```python
from build123d import *

# Parameters (mm, degrees)
SKETCH1_W                      = 68
SKETCH1_H                      = 68
SKETCH1_R                      = 14.29
BOSS_EXTRUDE1_DEPTH            = 10
M6_CLEARANCE_HOLE1_D           = 6.6
M6_CLEARANCE_HOLE1_CSINK_D     = 6.65
M6_CLEARANCE_HOLE1_CSINK_ANGLE = 100
SKETCH5_W                      = 120
SKETCH5_H                      = 10
BOSS_EXTRUDE3_DEPTH            = 68
M6_CLEARANCE_HOLE2_D           = 6.6
M6_CLEARANCE_HOLE2_CSINK_D     = 6.65
M6_CLEARANCE_HOLE2_CSINK_ANGLE = 100


with BuildPart() as part:
    # Sketch1 → Boss-Extrude1 (new body)
    with BuildSketch(Plane.XY):
        Rectangle(SKETCH1_W, SKETCH1_H)
        Circle(SKETCH1_R, mode=Mode.SUBTRACT)
    extrude(amount=BOSS_EXTRUDE1_DEPTH)

    # M6 Clearance Hole1 (through all)
    with Locations(Plane(origin=(0, 0, 0), x_dir=(-1, 0, 0), z_dir=(0, 0, -1))):
        with Locations((-18.768735293, 18.768735293), (18.768735293, 18.768735293), (-18.768735293, -18.768735293), (18.768735293, -18.768735293)):
            CounterSinkHole(M6_CLEARANCE_HOLE1_D / 2, M6_CLEARANCE_HOLE1_CSINK_D / 2, counter_sink_angle=M6_CLEARANCE_HOLE1_CSINK_ANGLE)

    # Sketch5 → Boss-Extrude3 (add)
    with BuildSketch(Plane.XY.offset(10)):
        with Locations((0, 29)):
            Rectangle(SKETCH5_W, SKETCH5_H)
    extrude(amount=BOSS_EXTRUDE3_DEPTH)

    # M6 Clearance Hole2 (through all)
    with Locations(Plane(origin=(0, 34, 0), x_dir=(1, 0, 0), z_dir=(0, 1, 0))):
        with Locations((-30, -24), (30, -24), (-30, -64), (30, -64)):
            CounterSinkHole(M6_CLEARANCE_HOLE2_D / 2, M6_CLEARANCE_HOLE2_CSINK_D / 2, counter_sink_angle=M6_CLEARANCE_HOLE2_CSINK_ANGLE)


solid = part.part
```
The listing builds one solid part. Answer for the finished solid, in the listing's coordinates (mm). A direction names the side the tool comes from. Round coordinates to 2 decimals unless told otherwise and drop trailing zeros. Loops run counter-clockwise (first coordinate to the right, second up) from the corner with the lowest first, then second, coordinate; pieces in that order, holes last. Notation, with made-up numbers: (65.5, 40.5) - (120.5, 40.5) arc R16 cw to (120.5, 50.5) - close; hole circle Ø11 at (34.25, 19). An arc over 180 degrees is marked (long way). Use one line per item in the form item = value. Start each with the question number.
1. The part is cut by section C-C on x = 0. Determine the outline of the cut face in (y, z).
2. The part is cut by section A-A on z = 24. Determine the outline of the cut face in (x, y) (3 decimals), then the cut area to 3 significant figures.
3. For a pull along X with two mould halves and no side action, classify faces 1 (the face through (28.226, 28.92, 61.217)), 2 (the face through (-1, 29, 78)), 3 (the face through (-60, 29, 44)) as pulls with the +X half, pulls with the -X half, needs draft (parallel to the pull), parting line crosses it, or undercut.
4. Given pin 1 Ø3 at (x, z) = (-15, 68.5) entering from -Y; pin 2 Ø4 at (x, z) = (-30, 24) entering from +Y; pin 3 Ø10 at (x, y) = (12, 6) entering from +Z; pin 4 Ø8 at (y, z) = (-12.5, 6.5) entering from +X, each flat-ended and moving along its own axis, determine where each tip first touches the part or whether it passes through.
5. Consider line 1 (Z direction, x = -30, y = 30.5); line 2 (X direction, y = 29.5, z = 24); line 3 (Y direction, x = -6, z = 37). Determine where each line is inside the solid, lowest interval first. Write a range as [from, to].
6. A tool of negligible diameter and unlimited length cuts with its end or side. For faces 4 (the face through (47, 29, 10)), 5 (the face through (15.47, 18.91, 5.08)), 6 (the face through (0, -17, 10)), 7 (the face through (0, -34, 5)), 8 (the face through (-47, 29, 10)), from which of +Z, -Z, +X, -X, +Y, -Y can it reach the whole face along a straight path? Write none if from no direction.
7. The part is cut by section B-B on x = -30. Determine the outline of the cut face in (y, z) (3 decimals).
8. The part is cut by section D-D on z = 47. Determine the outline of the cut face in (x, y), then the cut area to 3 significant figures.
Geometry check:
q1.outline = (-34, 0) - (-14.29, 0) - (-14.29, 10) - (-34, 10) - close; (14.29, 0) - (34, 0) - (34, 78) - (24, 78) - (24, 10) - (14.29, 10) - close
q2.outline = (-60, 24) - (-33.3, 24) - (-33.3, 33.979) - (-33.325, 34) - (-60, 34) - close; (-26.7, 24) - (26.7, 24) - (26.7, 33.979) - (26.675, 34) - (-26.675, 34) - (-26.7, 33.979) - close; (33.3, 24) - (60, 24) - (60, 34) - (33.325, 34) - (33.3, 33.979) - close
q2.area = 1,070 mm^2
q3.face_1 = undercut
q3.face_2 = needs draft
q3.face_3 = pulls with the -X half
q4.pin_1 = 24
q4.pin_2 = through
q4.pin_3 = 10
q4.pin_4 = 34
q5.line_1 = [0, 20.7], [27.3, 60.7], [67.3, 78]
q5.line_2 = [-60, -33.3], [-26.7, 26.7], [33.3, 60]
q5.line_3 = [24, 34]
q6.face_4 = -Z, +X, +Y, -Y
q6.face_5 = +Z, -Z
q6.face_6 = +Z, +X, -X, -Y
q6.face_7 = +Z, -Z, +X, -X, -Y
q6.face_8 = -Z, -X, +Y, -Y
q7.outline = (-34, 0) - (34, 0) - (34, 20.675) - (33.979, 20.7) - (24, 20.7) - (24, 10) - (-34, 10) - close; (24, 27.3) - (33.979, 27.3) - (34, 27.325) - (34, 60.675) - (33.979, 60.7) - (24, 60.7) - close; (24, 67.3) - (33.979, 67.3) - (34, 67.325) - (34, 78) - (24, 78) - close
q8.outline = (-60, 24) - (60, 24) - (60, 34) - (-60, 34) - close
q8.area = 1,200 mm^2
